```python
from build123d import *

# Parameters (mm, degrees)
BOSS_EXTRUDE1_DEPTH = 4
FILLET1_R           = 2
SKETCH2_R           = 0.75
CUT_EXTRUDE1_DEPTH  = 46
SKETCH4_W           = 10
SKETCH4_H           = 3
BOSS_EXTRUDE2_DEPTH = 4
SKETCH6_W           = 2
SKETCH6_H           = 10
BOSS_EXTRUDE3_DEPTH = 5


with BuildPart() as part:
    # Sketch1 → Boss-Extrude1 (new body)
    with BuildSketch(Plane(origin=(0, 0, 0), x_dir=(1, 0, 0), z_dir=(0, 1, 0))):
        with BuildLine():
            Line((-1, 23), (-1, -23))
            Line((-1, -23), (-40, -23))
            ThreePointArc((-40, -23), (-42.121320344, -22.121320344), (-43, -20))
            Line((-43, -20), (-43, 20))
            ThreePointArc((-43, 20), (-42.121320344, 22.121320344), (-40, 23))
            Line((-40, 23), (-1, 23))
        make_face()
    extrude(amount=BOSS_EXTRUDE1_DEPTH)

    # Fillet1
    fillet1_edges = [part.edges().sort_by_distance(p)[0] for p in [
        (-1, 0, 0),
        (-1, 4, 0),
    ]]
    fillet(fillet1_edges, radius=FILLET1_R - 0.0001)  # a hair under: the kernel refuses the full size

    # Sketch2 → Cut-Extrude1 (cut)
    with BuildSketch(Plane.XY.offset(23)):
        with Locations((-3, 2)):
            Circle(SKETCH2_R)
    extrude(amount=-CUT_EXTRUDE1_DEPTH, mode=Mode.SUBTRACT)

    # Sketch4 → Boss-Extrude2 (add)
    with BuildSketch(Plane.ZY.offset(43)):
        with Locations((0, 2.5)):
            Rectangle(SKETCH4_W, SKETCH4_H)
    extrude(amount=BOSS_EXTRUDE2_DEPTH)

    # Sketch6 → Boss-Extrude3 (add)
    with BuildSketch(Plane.XZ.offset(-1)):
        with Locations((-46, 0)):
            Rectangle(SKETCH6_W, SKETCH6_H)
    extrude(amount=BOSS_EXTRUDE3_DEPTH)


solid = part.part
```
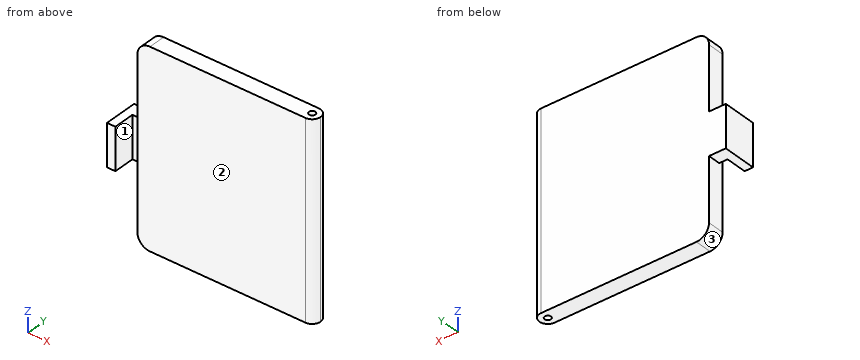
The listing builds one solid part. Answer for the finished solid, in the listing's coordinates (mm). Face numbers are marked on the shaded views. Coordinates: 2 decimals unless noted, no trailing zeros. Loops run counter-clockwise (first coordinate to the right, second up) from the corner with the lowest first, then second, coordinate; pieces in that order, holes last. Notation, with made-up numbers: M 82,52 L 91,52 A15 ccw 91,74 Z; hole C -25.5,45 d4. An arc over 180 degrees is marked long. Answer as a JSON object with one key per item and string values. Group by question number.
Item 1: Consider L1, parallel to Y at x = -3, z = -3; L2, parallel to Y at x = -11, z = -11; L3, parallel to Z at x = -44, y = 2. Determine where each line is inside the solid, lowest interval first.
Item 2: Section C-C (y = -2) is taken. Write down the section's boundary in (x, z), and give its area (3 significant figures).
Item 3: Each of these flat-tipped pins is pushed along its axis until it touches: P1, Ø2, axis at x = -45.5, y = 0.5, coming from the +Z side; P2, Ø12, axis at x = -12.5, z = -1, coming from the -Y side; P3, Ø4, axis at y = 1.5, z = -14.5, coming from the -X side. Where does it stop, or does it pass through?
Item 4: Section D-D (x = -32.5) is taken. Write down the section's boundary in (y, z).
Item 5: Determine the mould class of the marked faces 1, 2 and 3 for opening direction X: +X half, -X half, draft (parallel to the pull), parting line (faces both ways), or undercut.
Solved:
{
 "1": {"L1": "y = 0 to 1.25, 2.75 to 4", "L2": "y = 0 to 4", "L3": "z = -5 to 5"},
 "2": {"outline": "M -47,-5 L -45,-5 L -45,5 L -47,5 Z", "area": "20.0 mm2"},
 "3": {"P1": "stops at z = 5", "P2": "stops at y = 0", "P3": "stops at x = -43"},
 "4": {"outline": "M 0,-23 L 4,-23 L 4,23 L 0,23 Z"},
 "5": {"face 1": "undercut", "face 2": "draft", "face 3": "-X half"}
}
